Could you check a few things on this model? Use its own coordinates, in mm. Give positions to 0.01 mm unless a question says otherwise; leave off trailing zeros. Loops run counter-clockwise (first coordinate to the right, second up) from the corner with the lowest first, then second, coordinate; pieces in that order, holes last. Notation, with made-up numbers: M 43.5,7 L 74.5,7 A11 ccw 74.5,12 Z; hole C 45.25,-23.5 d7. An arc over 180 degrees is marked long. Return JSON: item names as keys, results as strings. Group by question number.
1. For pin 1 (1 mm diameter, centred on x = 21.5, z = 0.5, fed in from -Y); pin 2 (2.5 mm diameter, centred on x = 27.18, y = 10.06, fed in from -Z); pin 3 (1 mm diameter, centred on x = -9, z = 1.5, fed in from +Y), each with a flat end and sliding along its axis, tell me the tip position at first contact or that it passes through.
2. If we section it at B-B (x = 1): Write out the boundary of the cut face in (y, z), plus the area to 3 significant figures.
3. Please list where these lines run through material, in increasing order: line 1 (X direction, y = -10.5, z = 0.4); line 2 (Y direction, x = 15.5, z = 1.85); line 3 (X direction, y = -13.5, z = 1.65).
4. If we section it at A-A (y = 28): Write out the boundary of the cut face in (x, z), plus the area to 3 significant figures.
5. If we section it at D-D (y = 0): Write out the boundary of the cut face in (x, z), plus the area to 3 significant figures.
6. If we section it at C-C (x = 25.5): State how many separate pieces and enclosed holes the cut face has, plus the area to 3 significant figures.
```python
from build123d import *

# Parameters (mm, degrees)
F0_R     = 33
F1_DEPTH = 2
F3_DEPTH = 2.001
F5_DEPTH = 2.0010001
F6_R     = 0.7224908552
F6_R_2   = 0.7400457382
F7_DEPTH = 2.0010001


with BuildPart() as f1:
    # F0 (on Top) → F1 (new body)
    with BuildSketch(Plane.XY):
        Circle(F0_R)
    extrude(amount=F1_DEPTH)

    # F2 (on face) → F3 (cut, through all)
    with BuildSketch(Plane.XY.offset(2)):
        with BuildLine():
            ThreePointArc((26.6176071003, 14.1071927868), (22.716020238, 19.5321055237), (17.6763167755, 23.9199805513))
            ThreePointArc((17.6763167755, 23.9199805513), (-27.7198574863, 0), (17.6763167755, -23.9199805513))
            ThreePointArc((17.6763167755, -23.9199805513), (22.716020238, -19.5321055237), (26.6176071003, -14.1071927868))
            add(Edge.make_bspline(
                [(24.4190643431, -9.5471604607), (24.2953095849, -11.0698888291), (26.490861777, -12.1669797839), (26.6176071003, -14.1071927868)],
                knots=[0, 0, 0, 0, 0.3817701134, 0.3817701134, 0.3817701134, 0.3817701134], degree=3))
            Line((24.4190643431, -9.5471604607), (26.5364420049, -6.540675446))
            Line((26.5364420049, -6.540675446), (29.0613579283, -8.3188983701))
            ThreePointArc((29.0613579283, -8.3188983701), (29.97382864, -4.203852577), (30.2801425137, 0))
            ThreePointArc((30.2801425137, 0), (29.97382864, 4.203852577), (29.0613579283, 8.3188983701))
            Line((29.0613579283, 8.3188983701), (26.5364420049, 6.540675446))
            Line((26.5364420049, 6.540675446), (24.4190643431, 9.5471604607))
            add(Edge.make_bspline(
                [(24.4190643431, 9.5471604607), (24.2953095849, 11.0698888291), (26.490861777, 12.1669797839), (26.6176071003, 14.1071927868)],
                knots=[0, 0, 0, 0, 0.3817701134, 0.3817701134, 0.3817701134, 0.3817701134], degree=3))
        make_face()
    extrude(amount=-F3_DEPTH, mode=Mode.SUBTRACT)

    # F4 (on face) → F5 (cut, through all)
    with BuildSketch(Plane.XY.offset(2)):
        Polygon((31.331487748, 10.3603993888), (29.0613579283, 8.3188983701), (29.0613579283, -8.3188983701), (31.4715985336, -9.9266553149), (41.9540777802, 0), align=None)
    extrude(amount=-F5_DEPTH, mode=Mode.SUBTRACT)

    # F6 (on face) → F7 (cut, through all)
    with BuildSketch(Plane.XY.offset(2)):
        with Locations((27.1840710193, 10.0614046678)):
            Circle(F6_R)
        with Locations((27.2254403681, -9.8374607041)):
            Circle(F6_R_2)
    extrude(amount=-F7_DEPTH, mode=Mode.SUBTRACT)


solid = f1.part
```
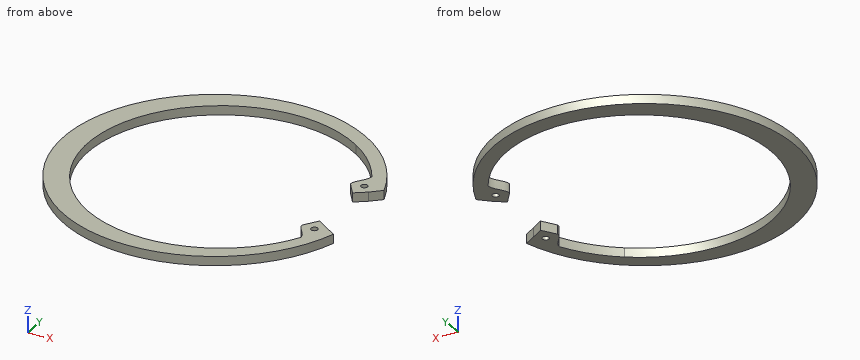
Answer:
{
 "1": {"pin 1": "stops at y = -25.46", "pin 2": "stops at z = 0", "pin 3": "stops at y = 31.89"},
 "2": {"outline": "M -32.98,0 L -29,0 L -29,2 L -32.98,2 Z; M 29,0 L 32.98,0 L 32.98,2 L 29,2 Z", "area": "15.9 mm²"},
 "3": {"line 1": "x = -31.28 to -25.75, 24.63 to 26.9, 27.56 to 31.28", "line 2": "y = -29.13 to -25.27, 25.27 to 29.13", "line 3": "x = -30.11 to -24.39, 26.51 to 30.11"},
 "4": {"outline": "M -17.46,0 L -6.27,0 L -6.27,2 L -17.46,2 Z; M 8.83,0 L 17.46,0 L 17.46,2 L 8.83,2 Z", "area": "39.7 mm²"},
 "5": {"outline": "M -33,0 L -27.72,0 L -27.72,2 L -33,2 Z", "area": "10.6 mm²"},
 "6": {"separate pieces": "4", "enclosed holes": "0", "area": "35.0 mm²"}
}
